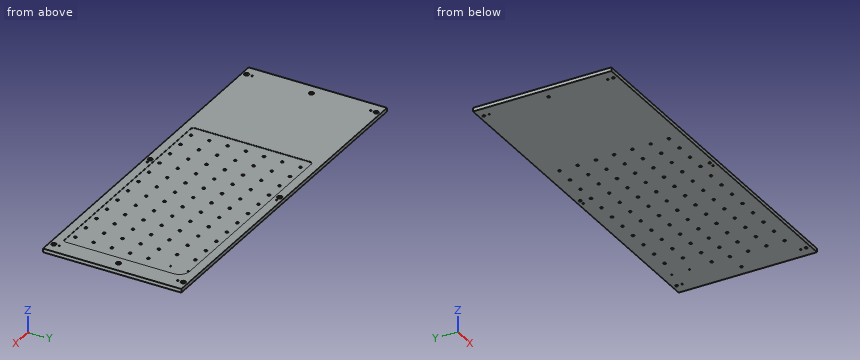
```python
from build123d import *

# Parameters (mm, degrees)
BOSS_EXTRUDE1_DEPTH                             = 10
CSK_FOR_M6_FLAT_HEAD_MACHINE_SCREW1_D           = 7
CSK_FOR_M6_FLAT_HEAD_MACHINE_SCREW1_CSINK_D     = 12.6
CSK_FOR_M6_FLAT_HEAD_MACHINE_SCREW1_CSINK_ANGLE = 90
CUT_EXTRUDE1_DEPTH                              = 0.5
M4X0_7_TAPPED_HOLE1_D                           = 3.3
M8X1_0_TAPPED_HOLE1_D                           = 7
LPATTERN1_COUNT                                 = 11
LPATTERN1_PITCH                                 = 50
LPATTERN1_COUNT_DIR2                            = 2
LPATTERN1_PITCH_DIR2                            = 50
M8X1_0_TAPPED_HOLE2_D                           = 7
LPATTERN2_COUNT                                 = 12
LPATTERN2_PITCH                                 = 50
LPATTERN2_COUNT_DIR2                            = 5
LPATTERN2_PITCH_DIR2                            = 50
M5X0_8_TAPPED_HOLE1_D                           = 4.2


with BuildPart() as part:
    # Sketch1 → Boss-Extrude1 (new body)
    with BuildSketch(Plane.XY):
        Polygon((-421, -145), (-421, -524), (-171, -524), (428, -524), (489, -524), (489, -492), (489, -177), (489, -145), (428, -145), (-171, -145), align=None)
        Polygon((-489, -177), (-489, -492), (-489, -524), (-421, -524), (-421, -145), (-489, -145), align=None)
    extrude(amount=BOSS_EXTRUDE1_DEPTH)

    # CSK for M6 Flat Head Machine Screw1 (through all)
    with Locations(Plane(origin=(458.5, -157, 10), x_dir=(1, 0, 0), z_dir=(0, 0, 1))):
        with Locations((0, 0), (0, -177.5), (0, -355), (-917, 0), (-917, -177.5), (-917, -355), (-458.5, 0), (-458.5, -355)):
            CounterSinkHole(CSK_FOR_M6_FLAT_HEAD_MACHINE_SCREW1_D / 2, CSK_FOR_M6_FLAT_HEAD_MACHINE_SCREW1_CSINK_D / 2, counter_sink_angle=CSK_FOR_M6_FLAT_HEAD_MACHINE_SCREW1_CSINK_ANGLE)

    # Sketch7 → Cut-Extrude1 (cut)
    with BuildSketch(Plane.XY.offset(10)):
        with BuildLine():
            Line((-179, -177), (-179, -492))
            ThreePointArc((-179, -492), (-176.656854249, -497.656854249), (-171, -500))
            Line((-171, -500), (428, -500))
            ThreePointArc((428, -500), (433.656854249, -497.656854249), (436, -492))
            Line((436, -492), (436, -197))
            ThreePointArc((436, -197), (427.798989873, -177.201010127), (408, -169))
            Line((408, -169), (-171, -169))
            ThreePointArc((-171, -169), (-176.656854249, -171.343145751), (-179, -177))
        make_face()
    extrude(amount=-CUT_EXTRUDE1_DEPTH, mode=Mode.SUBTRACT)

    # M4x0.7 Tapped Hole1 (through all)
    with Locations(Plane(origin=(408, -173, 9.5), x_dir=(1, 0, 0), z_dir=(0, 0, 1))):
        with Locations((0, 0), (0, -48)):
            Hole(M4X0_7_TAPPED_HOLE1_D / 2)

    # M8x1.0 Tapped Hole1 (through all)
    with Locations(Plane(origin=(-146.5, -184.5, 9.5), x_dir=(1, 0, 0), z_dir=(0, 0, 1))):
        with Locations((0, 0)):
            m8x1_0_tapped_hole1 = Hole(M8X1_0_TAPPED_HOLE1_D / 2)

    # LPattern1: M8x1.0 Tapped Hole1 11 × 2
    with Locations(*[(i * LPATTERN1_PITCH, -j * LPATTERN1_PITCH_DIR2, 0) for i in range(LPATTERN1_COUNT) for j in range(LPATTERN1_COUNT_DIR2) if (i, j) != (0, 0)]):
        add(m8x1_0_tapped_hole1, mode=Mode.SUBTRACT)

    # M8x1.0 Tapped Hole2 (through all)
    with Locations(Plane(origin=(-146.5, -484.5, 9.5), x_dir=(1, 0, 0), z_dir=(0, 0, 1))):
        with Locations((0, 0)):
            m8x1_0_tapped_hole2 = Hole(M8X1_0_TAPPED_HOLE2_D / 2)

    # LPattern2: M8x1.0 Tapped Hole2 12 × 5
    with Locations(*[(i * LPATTERN2_PITCH, j * LPATTERN2_PITCH_DIR2, 0) for i in range(LPATTERN2_COUNT) for j in range(LPATTERN2_COUNT_DIR2) if (i, j) != (0, 0)]):
        add(m8x1_0_tapped_hole2, mode=Mode.SUBTRACT)

    # M5x0.8 Tapped Hole1 (through all)
    with Locations(Plane(origin=(-458.5, -497, 10), x_dir=(1, 0, 0), z_dir=(0, 0, 1))):
        with Locations((0, 0), (0, 325), (917, 325), (917, 0), (473.5, 340), (473.5, -15)):
            Hole(M5X0_8_TAPPED_HOLE1_D / 2)


solid = part.part
```
Build history of the part. All positions in model axes, mm. Give positions to 0.01 mm unless a question says otherwise; leave off trailing zeros. Loops run counter-clockwise (first coordinate to the right, second up) from the corner with the lowest first, then second, coordinate; pieces in that order, holes last. Notation, with made-up numbers: (69, 79.5) - (121, 79.5) arc R34 cw to (121, 109.5) - close; hole circle Ø7 at (-6, -17.75). An arc over 180 degrees is marked (long way). Use a Markdown table: item, result.
(1) Band-saw the part on B-B (x = 82.5). Give the cut face in (y, z).
Taken from the geometry:
| item | result |
|---|---|
| outline | (-524, 0) - (-145, 0) - (-145, 10) - (-169, 10) - (-169, 9.5) - (-500, 9.5) - (-500, 10) - (-524, 10) - close |
(2) Wall check: line 1 along Y through (x, z) = (403.5, 5); line 2 along X through (y, z) = (-172, 3.5); line 3 along Z through (x, y) = (194.5, -488). Give the ranges that are in metal, low to high.
Taken from the geometry:
| item | result |
|---|---|
| line 1 | -524 to -488, -481 to -438, -431 to -388, -381 to -338, -331 to -288, -281 to -145 |
| line 2 | -489 to -460.6, -456.4 to 406.69, 409.31 to 456.4, 460.6 to 489 |
| line 3 | 0 to 9.5 |
(3) Drop flat-ended pins along their axis: pin 1 Ø8 at (x, y) = (303.5, -284.5) entering from +Z; pin 2 Ø8 at (x, y) = (458.5, -157) entering from +Z. Give the stop position or say it passes through.
Taken from the geometry:
| item | result |
|---|---|
| pin 1 | z = 9.5 |
| pin 2 | z = 7.7 |
(4) Band-saw the part on A-A (y = -267). Give the cut face in (x, z).
Taken from the geometry:
| item | result |
|---|---|
| outline | (-489, 0) - (489, 0) - (489, 10) - (436, 10) - (436, 9.5) - (-179, 9.5) - (-179, 10) - (-489, 10) - close |
